Source: CAD feature listing. Evaluate the final solid. Frame: model axes, mm. A direction names the side the tool comes from. Give positions to 0.01 mm unless a question says otherwise; leave off trailing zeros. Order: outer loops, then holes, each group sorted by start corner. A loop starts at its lowest first (then second) coordinate and runs counter-clockwise, first axis right, second up. Notation, with made-up numbers: (-39, -14) - (-19, -14) arc R9 cw to (-19, -6) - close; hole circle Ø5 at (21, 21). An arc over 180 degrees is marked (long way). Answer as CSV lines item,"result".
```python
from build123d import *

# Parameters (mm, degrees)
IZIM1_W                     = 80
IZIM1_H                     = 30
Y_KSEKLIK_EKSTR_ZYON1_DEPTH = 5
RADYUS2_R                   = 5
KES_EKSTR_ZYON1_DEPTH       = 8


with BuildPart() as part:
    # Çizim1 → Yükseklik-Ekstrüzyon1 (new body)
    with BuildSketch(Plane.XY):
        Rectangle(IZIM1_W, IZIM1_H)
    extrude(amount=Y_KSEKLIK_EKSTR_ZYON1_DEPTH)

    # Radyus2
    radyus2_edges = [part.edges().sort_by_distance(p)[0] for p in [
        (40, -15, 2.5),
        (-40, -15, 2.5),
    ]]
    fillet(radyus2_edges, radius=RADYUS2_R)

    # Çizim2 → Kes-Ekstrüzyon1 (cut)
    with BuildSketch(Plane.XY.offset(5)):
        with BuildLine():
            Line((-27.5, 4.1), (-12.5, 4.1))
            ThreePointArc((-12.5, 4.1), (-8.4, 0), (-12.5, -4.1))
            Line((-12.5, -4.1), (-27.5, -4.1))
            ThreePointArc((-27.5, -4.1), (-31.6, 0), (-27.5, 4.1))
        make_face()
        with BuildLine():
            Line((12.5, 4.1), (27.5, 4.1))
            ThreePointArc((27.5, 4.1), (31.6, 0), (27.5, -4.1))
            Line((27.5, -4.1), (12.5, -4.1))
            ThreePointArc((12.5, -4.1), (8.4, 0), (12.5, 4.1))
        make_face()
    extrude(amount=-KES_EKSTR_ZYON1_DEPTH, mode=Mode.SUBTRACT)


solid = part.part
```
(1) Mould query, pull axis X, two halves, no side actions, for faces 1 (the flat face through (20, -4.1, 3)), 2 (the flat face through (-40, 2, 2)), 3 (the flat face through (-1, 0, 0)). Classes: released by +X, released by -X, zero draft, split by the parting line, or undercut.
Completed:
face 1,"undercut"
face 2,"released by -X"
face 3,"zero draft"
(2) Cut plane C-C (z = 2.3). Return loops of the section in (x, y), then the cut area to 3 significant figures.
Completed:
outline,"(-40, -10) arc R5 ccw to (-35, -15) - (35, -15) arc R5 ccw to (40, -10) - (40, 15) - (-40, 15) - close; hole (-27.5, -4.1) - (-12.5, -4.1) arc R4.1 ccw to (-12.5, 4.1) - (-27.5, 4.1) arc R4.1 ccw to start; hole (12.5, -4.1) - (27.5, -4.1) arc R4.1 ccw to (27.5, 4.1) - (12.5, 4.1) arc R4.1 ccw to start"
area,"2,040 mm²"
(3) Cut plane A-A (y = 0). Return loops of the section in (x, z), then the cut area to 3 significant figures.
Completed:
outline,"(-40, 0) - (-31.6, 0) - (-31.6, 5) - (-40, 5) - close; (-8.4, 0) - (8.4, 0) - (8.4, 5) - (-8.4, 5) - close; (31.6, 0) - (40, 0) - (40, 5) - (31.6, 5) - close"
area,"168 mm²"
(4) Contact query for a flat-ended pin moving along its axis: pin 1 (1.5 mm diameter, centred on x = -9.5, y = 0.5, fed in from +Z). Output: stop coordinate, or through.
Completed:
pin 1,"through"
(5) Ray query, line 1 (X direction, y = 0.5, z = 3.4); line 2 (X direction, y = -3, z = 3); line 3 (Y direction, x = 16.5, z = 2.9). Return the intervals inside material, ascending. Write a range as from..to.
Completed:
line 1,"-40..-31.57, -8.43..8.43, 31.57..40"
line 2,"-40..-30.29, -9.71..9.71, 30.29..40"
line 3,"-15..-4.1, 4.1..15"
(6) Access query for faces 4 (the flat face through (40, 2, 2)), 5 (the cylindrical face through (8.4, -0.1, 2.5)). Directions: +Z, -Z, +X, -X, +Y, -Y. A direction counts if a zero-diameter tool reaches every point of the face in a straight line with its end or side. Return the directions, or none.
Completed:
face 4,"+Z, -Z, +X, +Y, -Y"
face 5,"+Z, -Z"
(7) Cut plane B-B (x = 23.5). Return loops of the section in (y, z), then the cut area to 3 significant figures.
Completed:
outline,"(-15, 0) - (-4.1, 0) - (-4.1, 5) - (-15, 5) - close; (4.1, 0) - (15, 0) - (15, 5) - (4.1, 5) - close"
area,"109 mm²"
